```python
from build123d import *

# Parameters (mm, degrees)
SKETCH1_W               = 75
SKETCH1_H               = 25
BOSS_EXTRUDE1_DEPTH     = 8
SKETCH5_W               = 25
SKETCH5_H               = 21
BOSS_EXTRUDE2_DEPTH     = 50
SKETCH7_W               = 16.7
SKETCH7_H               = 16.7
CUT_EXTRUDE3_DEPTH      = 45
SKETCH4_R               = 2.38125
CUT_EXTRUDE2_DEPTH      = 50.025503567
CUT_EXTRUDE1_DEPTH      = 45.760473635
CUT_EXTRUDE1_DEPTH_BACK = 5
SKETCH3_R               = 4
FILLET1_R               = 3
SKETCH8_R               = 3.175
CUT_EXTRUDE4_DEPTH      = 77.793554417


with BuildPart() as part:
    # Sketch1 → Boss-Extrude1 (new body)
    with BuildSketch(Plane(origin=(0, 0, 0), x_dir=(1, 0, 0), z_dir=(0, 1, 0))):
        Rectangle(SKETCH1_W, SKETCH1_H)
    extrude(amount=BOSS_EXTRUDE1_DEPTH)

    # Sketch5 → Boss-Extrude2 (add)
    with BuildSketch(Plane.ZY.offset(37.5)):
        with Locations((0, 18.5)):
            Rectangle(SKETCH5_W, SKETCH5_H)
    extrude(amount=-BOSS_EXTRUDE2_DEPTH)

    # Sketch7 → Cut-Extrude3 (cut)
    with BuildSketch(Plane(origin=(12.5, 0, 0), x_dir=(0, 0, -1), z_dir=(1, 0, 0))):
        with Locations((0, 16.35)):
            Rectangle(SKETCH7_W, SKETCH7_H)
    extrude(amount=-CUT_EXTRUDE3_DEPTH, mode=Mode.SUBTRACT)

    # Sketch4 → Cut-Extrude2 (cut, through all)
    with BuildSketch(Plane(origin=(0, 0, 0), x_dir=(1, 0, 0), z_dir=(0, 1, 0))):
        with Locations(Location((0, 0, 0), (0, 0, 90))):
            Circle(SKETCH4_R)
        with Locations(Location((25.4, 0, 0), (0, 0, 90))):
            Circle(SKETCH4_R)
        with Locations(Location((-25.4, 0, 0), (0, 0, 90))):
            Circle(SKETCH4_R)
    extrude(amount=CUT_EXTRUDE2_DEPTH, mode=Mode.SUBTRACT)

    # Sketch3 → Cut-Extrude1 (cut, two sides: drawn at the far end of the back side and taken through both)
    with BuildSketch(Plane(origin=(0, 8, 0), x_dir=(1, 0, 0), z_dir=(0, 1, 0)).offset(-CUT_EXTRUDE1_DEPTH_BACK)):
        with Locations(Location((0, 0, 0), (0, 0, 90))):
            Circle(SKETCH3_R)
        with Locations(Location((25.4, 0, 0), (0, 0, 90))):
            Circle(SKETCH3_R)
        with Locations(Location((-25.4, 0, 0), (0, 0, 90))):
            Circle(SKETCH3_R)
    extrude(amount=CUT_EXTRUDE1_DEPTH + CUT_EXTRUDE1_DEPTH_BACK, mode=Mode.SUBTRACT)

    # Fillet1
    fillet1_edges = [part.edges().sort_by_distance(p)[0] for p in [
        (25, 8, 12.5),
        (12.5, 18.5, -12.5),
        (12.5, 29, 0),
        (-12.5, 29, -12.5),
        (12.5, 18.5, 12.5),
        (-12.5, 29, 12.5),
        (12.5, 8, -10.425),
        (-37.5, 29, 0),
        (12.5, 8, 10.425),
        (37.5, 8, 0),
        (37.5, 4, 12.5),
        (-37.5, 14.5, 12.5),
        (-37.5, 14.5, -12.5),
        (37.5, 4, -12.5),
        (25, 8, -12.5),
    ]]
    fillet(fillet1_edges, radius=FILLET1_R)

    # Sketch8 → Cut-Extrude4 (cut, through all)
    with BuildSketch(Plane(origin=(-32.5, 0, 0), x_dir=(0, 0, -1), z_dir=(1, 0, 0))):
        with Locations((0, 16.35)):
            Circle(SKETCH8_R)
    extrude(amount=-CUT_EXTRUDE4_DEPTH, mode=Mode.SUBTRACT)


solid = part.part
```
Check sheet for the modelled part. Datum: model origin and axes. Units: mm. A direction names the side the tool comes from. Round coordinates to 2 decimals unless told otherwise and drop trailing zeros. Order: outer loops, then holes, each group sorted by start corner. A loop starts at its lowest first (then second) coordinate and runs counter-clockwise, first axis right, second up. Notation, with made-up numbers: (-25.5, -11.75) - (2.5, -11.75) arc R22 cw to (2.5, -2.75) - close; hole circle Ø3 at (32, 2.5). An arc over 180 degrees is marked (long way). Write item = value, one per line.
Q1. Thickness scan on line 1 along X through (y, z) = (4.6, 0); line 2 along Z through (x, y) = (-31.5, 21.5); line 3 along X through (y, z) = (1.5, -1). Record the ranges inside material, lowest first.
Computed:
line_1 = -37.5 to -29.4, -21.4 to -4, 4 to 21.4, 29.4 to 37.5
line_2 = -12.5 to -8.35, 8.35 to 12.5
line_3 = -37.5 to -27.56, -23.24 to -2.16, 2.16 to 23.24, 27.56 to 37.5
Q2. Section check C-C (z = -7.5). Record the boundary of the cut face in (x, y).
Computed:
outline = (-37.5, 0) - (37.5, 0) - (37.5, 5) arc R3 ccw to (34.5, 8) - (-32.5, 8) - (-32.5, 24.7) - (12.5, 24.7) - (12.5, 26) arc R3 ccw to (9.5, 29) - (-34.5, 29) arc R3 ccw to (-37.5, 26) - close
Q3. Section check B-B (y = 16.35). Record the boundary of the cut face in (x, z) (3 decimals).
Computed:
outline = (-37.5, -9.5) arc R3 ccw to (-34.5, -12.5) - (9.5, -12.5) arc R3 ccw to (12.5, -9.5) - (12.5, -8.35) - (-32.5, -8.35) - (-32.5, -3.175) - (-37.5, -3.175) - close; (-37.5, 3.175) - (-32.5, 3.175) - (-32.5, 8.35) - (12.5, 8.35) - (12.5, 9.5) arc R3 ccw to (9.5, 12.5) - (-34.5, 12.5) arc R3 ccw to (-37.5, 9.5) - close
Q4. Section check A-A (x = 25.4). Record the boundary of the cut face in (y, z), and give its area (3 significant figures).
Computed:
outline = (0, -12.5) - (5, -12.5) arc R3 ccw to (8, -9.5) - (8, -4) - (3, -4) - (3, -2.38) - (0, -2.38) - close; (0, 2.38) - (3, 2.38) - (3, 4) - (8, 4) - (8, 9.5) arc R3 ccw to (5, 12.5) - (0, 12.5) - close
area = 142 mm^2
Q5. Tool access check on faces 1 (the face through (-8, 13, 12.5)), 2 (the face through (-8, 16, 8.35)), 3 (the face through (2, 3, -2)). Record the directions out of +Z, -Z, +X, -X, +Y, -Y that give a thin tool (end or side, any length) a straight path to the whole face; none if there is none.
Computed:
face_1 = +Z, +X, -X, +Y, -Y
face_2 = +X
face_3 = +Y
Q6. Draft check along X on faces 4 (the face through (25.13, 7.14, 11.6)), 5 (the face through (27, 3, -2)), 6 (the face through (12.5, 25, -1)). Enter one of: pulls with the +X half, pulls with the -X half, needs draft (parallel to the pull), parting line crosses it, or undercut.
Computed:
face_4 = needs draft
face_5 = undercut
face_6 = pulls with the +X half
Q7. Go/stop test with flat-tipped pins: pin 1 (12 mm diameter, centred on x = 29.5, y = 17, fed in from +Z); pin 2 (13 mm diameter, centred on x = 25.4, z = 0, fed in from +Y); pin 3 (4 mm diameter, centred on x = 26, z = -0.5, fed in from +Y); pin 4 (8.5 mm diameter, centred on y = 13.5, z = -2.5, fed in from +X). Record where each tip stops, or that it passes through.
Computed:
pin_1 = through
pin_2 = 8
pin_3 = 3
pin_4 = -32.5
Q8. Section check D-D (x = -25.4). Record the boundary of the cut face in (y, z), and give its area (3 significant figures).
Computed:
outline = (0, -12.5) - (26, -12.5) arc R3 ccw to (29, -9.5) - (29, -4) - (24.7, -4) - (24.7, -8.35) - (8, -8.35) - (8, -4) - (3, -4) - (3, -2.38) - (0, -2.38) - close; (0, 2.38) - (3, 2.38) - (3, 4) - (8, 4) - (8, 8.35) - (24.7, 8.35) - (24.7, 4) - (29, 4) - (29, 9.5) arc R3 ccw to (26, 12.5) - (0, 12.5) - close
area = 354 mm^2
